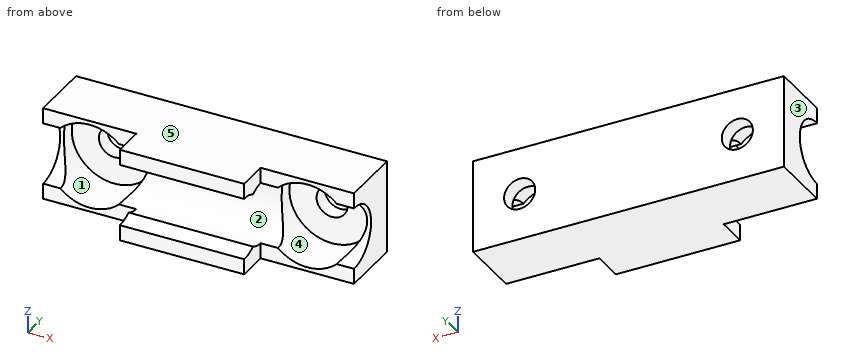
from build123d import *

# Parameters (mm, degrees)
CYLINDER042_R     = 5.5
CYLINDER042_DEPTH = 10
BOX012_W          = 12
BOX012_H          = 4
BOX012_DEPTH      = 12
CYLINDER041_R     = 2
CYLINDER041_DEPTH = 12
CYLINDER040_R     = 5.5
CYLINDER040_DEPTH = 10
BOX011_W          = 12
BOX011_H          = 4
BOX011_DEPTH      = 12
CYLINDER039_R     = 2
CYLINDER039_DEPTH = 12
CYLINDER043_R     = 4
CYLINDER043_DEPTH = 40
CYLINDER038_R     = 4
CYLINDER038_DEPTH = 40
BOX009_W          = 40
BOX009_H          = 12
BOX009_DEPTH      = 12


with BuildPart() as cylinder042:
    # Cylinder042 → Cylinder042 (new body)
    with BuildSketch(Plane(origin=(20, 10, 6), x_dir=(1, 0, 0), z_dir=(0, -1, 0))):
        Circle(CYLINDER042_R)
    extrude(amount=CYLINDER042_DEPTH)


with BuildPart() as cube012:
    # Box012 → Box012 (new body)
    with BuildSketch(Plane(origin=(14, 0, 0), x_dir=(1, 0, 0), z_dir=(0, 0, 1))):
        with Locations((6, 2)):
            Rectangle(BOX012_W, BOX012_H)
    extrude(amount=BOX012_DEPTH)


with BuildPart() as fusion014:
    # Cylinder041 → Cylinder041 (new body)
    with BuildSketch(Plane(origin=(20, 12, 6), x_dir=(1, 0, 0), z_dir=(0, -1, 0))):
        Circle(CYLINDER041_R)
    extrude(amount=CYLINDER041_DEPTH)

    # Fusion014: union Cylinder042, Cube012
    add(cylinder042.part)
    add(cube012.part)


with BuildPart() as fusion014_1:
    # Fusion014 placement: moved
    add(fusion014.part.moved(Location((14, 0, 0))))


with BuildPart() as cylinder040:
    # Cylinder040 → Cylinder040 (new body)
    with BuildSketch(Plane(origin=(20, 10, 6), x_dir=(1, 0, 0), z_dir=(0, -1, 0))):
        Circle(CYLINDER040_R)
    extrude(amount=CYLINDER040_DEPTH)


with BuildPart() as cube011:
    # Box011 → Box011 (new body)
    with BuildSketch(Plane(origin=(14, 0, 0), x_dir=(1, 0, 0), z_dir=(0, 0, 1))):
        with Locations((6, 2)):
            Rectangle(BOX011_W, BOX011_H)
    extrude(amount=BOX011_DEPTH)


with BuildPart() as fusion015:
    # Cylinder039 → Cylinder039 (new body)
    with BuildSketch(Plane(origin=(20, 12, 6), x_dir=(1, 0, 0), z_dir=(0, -1, 0))):
        Circle(CYLINDER039_R)
    extrude(amount=CYLINDER039_DEPTH)

    # Fusion013: union Cylinder040, Cube011
    add(cylinder040.part)
    add(cube011.part)


with BuildPart() as fusion015_1:
    # Fusion013 placement: moved
    add(fusion015.part.moved(Location((-14, 0, 0))))

    # Fusion015: union Fusion014
    add(fusion014_1.part)


with BuildPart() as cylinder043:
    # Cylinder043 → Cylinder043 (new body)
    with BuildSketch(Plane(origin=(0, 0.15, 6), x_dir=(0, 0, -1), z_dir=(1, 0, 0))):
        Circle(CYLINDER043_R)
    extrude(amount=CYLINDER043_DEPTH)


with BuildPart() as fusion016:
    # Cylinder038 → Cylinder038 (new body)
    with BuildSketch(Plane(origin=(0, 4.15, 6), x_dir=(0, 0, -1), z_dir=(1, 0, 0))):
        Circle(CYLINDER038_R)
    extrude(amount=CYLINDER038_DEPTH)

    # Fusion016: union Cylinder043
    add(cylinder043.part)


with BuildPart() as cut015:
    # Box009 → Box009 (new body)
    with BuildSketch(Plane.XY):
        with Locations((20, 6)):
            Rectangle(BOX009_W, BOX009_H)
    extrude(amount=BOX009_DEPTH)

    # Cut014: cut Fusion016
    add(fusion016.part, mode=Mode.SUBTRACT)

    # Cut015: cut Fusion015
    add(fusion015_1.part, mode=Mode.SUBTRACT)


solid = cut015.part
The model under review builds one solid part; all positions refer to its coordinate system, in mm. Face numbers are marked on the shaded views. A direction names the side the tool comes from. Coordinates: 2 decimals unless noted, no trailing zeros. Loops run counter-clockwise (first coordinate to the right, second up) from the corner with the lowest first, then second, coordinate; pieces in that order, holes last. Notation, with made-up numbers: (-13, -4) -> (33, -4) arc R9 cw to (33, 0) -> close; hole circle Ø3 at (-31.75, 10). An arc over 180 degrees is marked (long way). Use a Markdown table: item, result. Add a question column.
1. Add section D-D on x = 22. Write out the cut boundary in (y, z), plus the area to 3 significant figures.
2. Machinability: for the marked faces 1 and 2, which of the approach directions +Z, -Z, +X, -X, +Y, -Y give a long, thin tool a straight path to every point of the face, cutting with its end or side? Answer none if there is none.
3. Add section C-C on y = 9.5. Write out the cut boundary in (x, z), plus the area to 3 significant figures.
4. Clearance check with flat-ended pins moving along their axes: pin 1 Ø1 at (x, z) = (7.5, 8) entering from -Y; pin 2 Ø0.8 at (y, z) = (2.5, 1.5) entering from +X; pin 3 Ø1.6 at (x, z) = (6, 0.5) entering from -Y. State where each tip first meets the part, or that it passes through.
5. Add section B-B on z = 6. Write out the cut boundary in (x, y), plus the area to 3 significant figures.
6. To check wall thickness, follow line 1 (Z direction, x = 6, y = 10.95); line 2 (X direction, y = 8.5, z = 6); line 3 (Z direction, x = 15.5, y = 4.15). State the ranges of each line that lie inside material, in increasing order.
7. Add section A-A on x = 6. Write out the cut boundary in (y, z), plus the area to 3 significant figures.
8. Draft analysis for pull direction Z (two halves, no side actions). For the marked faces 3, 4 and 5, state which applies: pulls with the +Z half, pulls with the -Z half, needs draft (parallel to the pull), parting line crosses it, or undercut.
Returned:
| question | item | result |
|---|---|---|
| 1 | outline | (0, 0) -> (12, 0) -> (12, 12) -> (0, 12) -> (0, 10) arc R4 cw to (2.15, 9.46) arc R4 cw (long way) to (2.15, 2.54) arc R4 cw to (0, 2) -> close |
| 1 | area | 87.1 mm² |
| 2 | face 1 | -Y |
| 2 | face 2 | +X, -X |
| 3 | outline | (0, 0) -> (40, 0) -> (40, 12) -> (0, 12) -> close; hole circle Ø11 at (6, 6); hole circle Ø11 at (34, 6) |
| 3 | area | 290 mm² |
| 4 | pin 1 | stops at y = 10 |
| 4 | pin 2 | stops at x = 28 |
| 4 | pin 3 | stops at y = 4 |
| 5 | outline | (0, 8.15) -> (0.5, 8.15) -> (0.5, 10) -> (4, 10) -> (4, 12) -> (0, 12) -> close; (8, 10) -> (11.5, 10) -> (11.5, 8.15) -> (28.5, 8.15) -> (28.5, 10) -> (32, 10) -> (32, 12) -> (8, 12) -> close; (36, 10) -> (39.5, 10) -> (39.5, 8.15) -> (40, 8.15) -> (40, 12) -> (36, 12) -> close |
| 5 | area | 97.3 mm² |
| 6 | line 1 | z = 0 to 4, 8 to 12 |
| 6 | line 2 | x = 0 to 0.5, 11.5 to 28.5, 39.5 to 40 |
| 6 | line 3 | z = 0 to 2, 10 to 12 |
| 7 | outline | (4, 0) -> (12, 0) -> (12, 4) -> (10, 4) -> (10, 0.5) -> (4, 0.5) -> close; (4, 11.5) -> (10, 11.5) -> (10, 8) -> (12, 8) -> (12, 12) -> (4, 12) -> close |
| 7 | area | 22.0 mm² |
| 8 | face 3 | needs draft |
| 8 | face 4 | undercut |
| 8 | face 5 | pulls with the +Z half |
